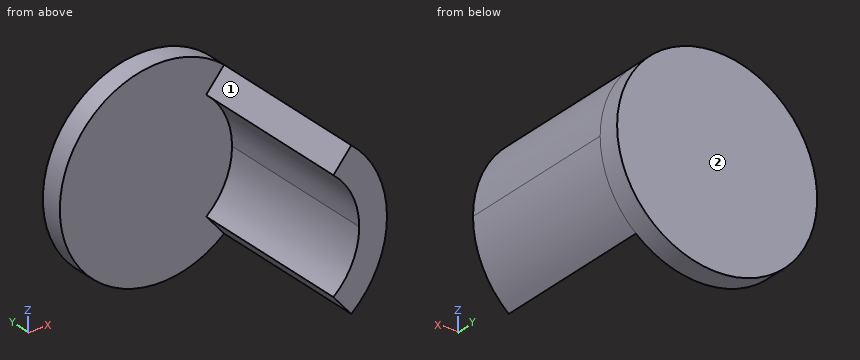
```python
from build123d import *

# Parameters (mm, degrees)
SKIZZE1_R                       = 18
AUFSATZ_LINEAR_AUSTRAGEN1_DEPTH = 4
AUFSATZ_LINEAR_AUSTRAGEN2_DEPTH = 30


with BuildPart() as part:
    # Skizze1 → Aufsatz-Linear austragen1 (new body)
    with BuildSketch(Plane(origin=(0, 0, 0), x_dir=(1, 0, 0), z_dir=(0, 1, 0))):
        Circle(SKIZZE1_R)
    extrude(amount=AUFSATZ_LINEAR_AUSTRAGEN1_DEPTH)

    # Skizze2 → Aufsatz-Linear austragen2 (add)
    with BuildSketch(Plane.XZ):
        with BuildLine():
            Line((11.570176974, 13.788799976), (8.356238926, 9.958577761))
            ThreePointArc((8.356238926, 9.958577761), (11.782001231, 5.494037403), (13, 0))
            ThreePointArc((13, 0), (11.782001231, -5.494037403), (8.356238926, -9.958577761))
            Line((8.356238926, -9.958577761), (11.570176974, -13.788799976))
            ThreePointArc((11.570176974, -13.788799976), (16.313540167, -7.607128711), (18, 0))
            ThreePointArc((18, 0), (16.313540167, 7.607128711), (11.570176974, 13.788799976))
        make_face()
    extrude(amount=AUFSATZ_LINEAR_AUSTRAGEN2_DEPTH)


solid = part.part
```
Build history of the part. All positions in model axes, mm. Face numbers are marked on the shaded views. A direction names the side the tool comes from. Coordinates: 2 decimals unless noted, no trailing zeros. Order: outer loops, then holes, each group sorted by start corner. A loop starts at its lowest first (then second) coordinate and runs counter-clockwise, first axis right, second up.
Item 1: Saw through at D-D on y = -14. List the corners of the cut face in (x, z).
Filled in:
outline: (8.36, -9.96) - (11.57, -13.79) arc R18 ccw to (11.57, 13.79) - (8.36, 9.96) arc R13 cw to start
Item 2: Tool access for the marked faces 1 and 2: list every direction of +Z, -Z, +X, -X, +Y, -Y with a clear straight run to the whole face (end or side of a thin tool).
Filled in:
face 1: +Z, -X, -Y
face 2: +Z, -Z, +X, -X, +Y
Item 3: Drill centre lines: L1, parallel to Y at x = -7.5, z = -1; L2, parallel to Z at x = 9, y = -13.5; L3, parallel to Z at x = 12, y = -10.5. Where is each one in solid material? Low to high.
Filled in:
L1: y = 0 to 4
L2: z = -10.73 to -9.38, 9.38 to 10.73
L3: z = -13.42 to -5, 5 to 13.42
Item 4: Drop flat-ended pins along their axis: pin 1 Ø5 at (y, z) = (-1.5, -14) entering from -X; pin 2 Ø2 at (x, z) = (3, 13.5) entering from -Y; pin 3 Ø8 at (x, y) = (14.5, -21) entering from -Z. Give the stop position or say it passes through.
Filled in:
pin 1: stops at x = -13.42
pin 2: stops at y = 0
pin 3: stops at z = -13.79
Item 5: Saw through at C-C on x = 0. List the corners of the cut face in (y, z), then the cut area to 3 significant figures.
Filled in:
outline: (0, -18) - (4, -18) - (4, 18) - (0, 18) - close
area: 144 mm2
Item 6: Saw through at A-A on y = 0.5. List the corners of the cut face in (x, z), then the cut area to 3 significant figures.
Filled in:
outline: circle Ø36 at (0, 0)
area: 1,020 mm2
Item 7: Saw through at B-B on z = -13. List the corners of the cut face in (x, y).
Filled in:
outline: (-12.45, 0) - (10.91, 0) - (10.91, -30) - (12.45, -30) - (12.45, 4) - (-12.45, 4) - close
